Check sheet for the modelled part. Datum: model origin and axes. Units: mm. A direction names the side the tool comes from. Coordinates: 2 decimals unless noted, no trailing zeros. Write each loop counter-clockwise with the first axis right and the second up, starting at its lowest first coordinate (ties: lowest second). Pieces come first, ordered by that corner, then holes. Notation, with made-up numbers: (64.5, 21.5) - (90.5, 21.5) arc R30 ccw to (90.5, 43.5) - close; hole circle Ø3 at (80, 30). An arc over 180 degrees is marked (long way). Write each question's results on one line, items separated by ' | '.
from build123d import *

# Parameters (mm, degrees)
SKETCH2_W           = 140
SKETCH2_H           = 140
SKETCH2_W_2         = 120
SKETCH2_H_2         = 120
EXTRUDE_THIN1_DEPTH = 120
SKETCH3_W           = 140
SKETCH3_H           = 140
BOSS_EXTRUDE1_DEPTH = 10
CUT_EXTRUDE1_REACH  = 199.231
SKETCH5_R           = 53
CUT_EXTRUDE4_REACH  = 165.401


with BuildPart() as part:
    # Sketch2 → Extrude-Thin1 (new body)
    with BuildSketch(Plane(origin=(0, 0, 0), x_dir=(0, 0, -1), z_dir=(1, 0, 0))):
        Rectangle(SKETCH2_W, SKETCH2_H)
        Rectangle(SKETCH2_W_2, SKETCH2_H_2, mode=Mode.SUBTRACT)
    extrude(amount=EXTRUDE_THIN1_DEPTH)

    # Sketch3 → Boss-Extrude1 (add)
    with BuildSketch(Plane.ZY):
        Rectangle(SKETCH3_W, SKETCH3_H)
    extrude(amount=BOSS_EXTRUDE1_DEPTH)

    # Sketch5 → Cut-Extrude1 (cut, up to next)
    with BuildSketch(Plane(origin=(0, 70, 0), x_dir=(1, 0, 0), z_dir=(0, 1, 0)), mode=Mode.PRIVATE) as cut_extrude1_sk1:
        with Locations(Location((55, 0, 0), (0, 0, 270))):
            Circle(SKETCH5_R)
    cut_extrude1_tool1 = extrude(cut_extrude1_sk1.sketch, amount=-CUT_EXTRUDE1_REACH, mode=Mode.PRIVATE) & part.part
    add(cut_extrude1_tool1.solids().sort_by_distance((55, 70, 0))[0], mode=Mode.SUBTRACT)

    # Sketch8 → Cut-Extrude4 (cut, up to next)
    with BuildSketch(Plane.ZY.offset(10), mode=Mode.PRIVATE) as cut_extrude4_sk1:
        with BuildLine():
            Line((-25, 40), (25, 40))
            ThreePointArc((25, 40), (0, 15), (-25, 40))
        make_face()
    cut_extrude4_tool1 = extrude(cut_extrude4_sk1.sketch, amount=-CUT_EXTRUDE4_REACH, mode=Mode.PRIVATE) & part.part
    add(cut_extrude4_tool1.solids().sort_by_distance((-10, 29.38967, 0))[0], mode=Mode.SUBTRACT)


solid = part.part
1. Sectioned sample at D-D (z = 27.5). Record the cut outline in (x, y), then the cut area to 3 significant figures.
Values follow:
outline: (-10, -70) - (120, -70) - (120, -60) - (0, -60) - (0, 60) - (9.69, 60) - (9.69, 70) - (-10, 70) - close; (100.31, 60) - (120, 60) - (120, 70) - (100.31, 70) - close | area: 2,890 mm^2
2. Draft check along Z on faces 1 (the flat face through (-10, 1, -1)), 2 (the flat face through (112, 60, 1)), 3 (the flat face through (56, -1, 70)), 4 (the flat face through (56, -1, -70)). Enter one of: pulls with the +Z half, pulls with the -Z half, needs draft (parallel to the pull), parting line crosses it, or undercut.
Values follow:
face 1: needs draft | face 2: undercut | face 3: pulls with the +Z half | face 4: pulls with the -Z half
3. Sectioned sample at B-B (x = 55). Record the cut outline in (y, z), then the cut area to 3 significant figures.
Values follow:
outline: (-70, -70) - (70, -70) - (70, -53) - (60, -53) - (60, -60) - (-60, -60) - (-60, 60) - (60, 60) - (60, 53) - (70, 53) - (70, 70) - (-70, 70) - close | area: 4,140 mm^2
4. Sectioned sample at C-C (y = 5). Record the cut outline in (x, z), then the cut area to 3 significant figures.
Values follow:
outline: (-10, -70) - (120, -70) - (120, -60) - (0, -60) - (0, 60) - (120, 60) - (120, 70) - (-10, 70) - close | area: 3,800 mm^2
5. Sectioned sample at A-A (z = 0). Record the cut outline in (x, y).
Values follow:
outline: (-10, -70) - (120, -70) - (120, -60) - (0, -60) - (0, 15) - (-10, 15) - close; (-10, 40) - (0, 40) - (0, 60) - (2, 60) - (2, 70) - (-10, 70) - close; (108, 60) - (120, 60) - (120, 70) - (108, 70) - close
6. Access from +Z, -Z, +X, -X, +Y, -Y to the whole of each face (thin tool, end or side, straight path). Record for faces 5 (the flat face through (99, 70, -32)), 6 (the flat face through (-5, 40, 0)), 7 (the flat face through (56, -70, -1)), 8 (the flat face through (0, 1, -1)), 9 (the cylindrical face through (3.26, 65.07, -11.49)).
Values follow:
face 5: +Z, -Z, +X, -X, +Y | face 6: +X, -X | face 7: +Z, -Z, +X, -X, -Y | face 8: +X | face 9: +Y
7. Go/stop test with a flat-tipped pin: pin 1 (5 mm diameter, centred on x = 79, z = -28, fed in from +Y). Record where the tip stops, or that it passes through.
Values follow:
pin 1: stops at y = -60
8. Material ranges on L1, parallel to Z at x = 56, y = 14; L2, parallel to X at y = 67.25, z = 0; L3, parallel to Y at x = 98.5, z = -15, recorded low to high. Write a range as [from, to].
Values follow:
L1: z = [-70, -60], [60, 70] | L2: x = [-10, 2], [108, 120] | L3: y = [-70, -60]
